```python
from build123d import *

# Parameters (mm, degrees)
FILLET1_R      = 6
CHAMFER1_SIZE  = 1
CHAMFER1_SIZE2 = 2
CHAMFER2_SIZE  = 0.5


with BuildPart() as part:
    # Sketch1 → Revolve1 (revolve)
    with BuildSketch(Plane(origin=(0, 0, 0), x_dir=(0, 0, -1), z_dir=(1, 0, 0)), mode=Mode.PRIVATE) as revolve1_sk:
        Polygon((0, 0), (0, -78.067128988), (11, -78.067128988), (11, -75.067128988), (2.5, -75.067128988), (2.5, -8), (1.5, -8), (1.5, -3), (2.5, -3), (2.5, 0), align=None)
    revolve(revolve1_sk.sketch.rotate(Axis((0, 0, 0), (0, -1, 0)), 180), axis=Axis((0, 0, 0), (0, -1, 0)))

    # Fillet1
    fillet1_edges = [part.edges().sort_by_distance(p)[0] for p in [
        (0, -75.067128988, -2.5),
    ]]
    fillet(fillet1_edges, radius=FILLET1_R)

    # Chamfer1
    chamfer1_edges = [part.edges().sort_by_distance(p)[0] for p in [
        (0, -75.067128988, -11),
    ]]
    chamfer1_side = [part.faces().sort_by_distance(p)[0] for p in [
        (0, -76.567128988, -11),
    ]]
    chamfer(chamfer1_edges, length=CHAMFER1_SIZE, length2=CHAMFER1_SIZE2, reference=chamfer1_side[0])

    # Chamfer2
    chamfer2_edges = [part.edges().sort_by_distance(p)[0] for p in [
        (0, 0, -2.5),
    ]]
    chamfer(chamfer2_edges, length=CHAMFER2_SIZE)


solid = part.part
```
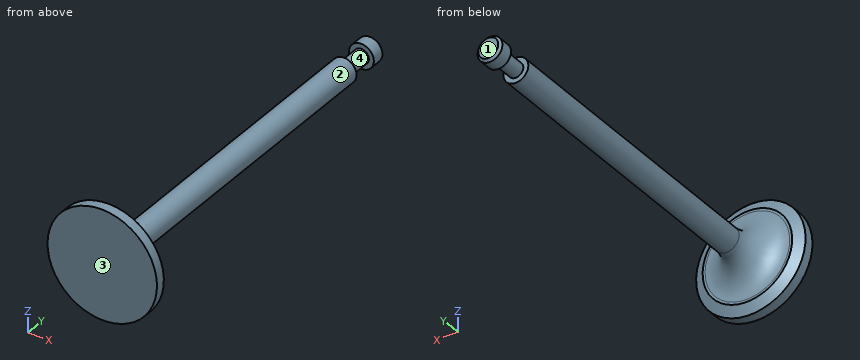
Build history of the part. All positions in model axes, mm. Face numbers are marked on the shaded views. Give positions to 0.01 mm unless a question says otherwise; leave off trailing zeros. Loops run counter-clockwise (first coordinate to the right, second up) from the corner with the lowest first, then second, coordinate; pieces in that order, holes last. Notation, with made-up numbers: (50.5, 36) - (85.5, 36) arc R21 ccw to (85.5, 75) - close; hole circle Ø10 at (58, 12). An arc over 180 degrees is marked (long way). Use a Markdown table: item, result.
(1) Band-saw the part on C-C (y = -50). Give the cut face in (x, z), and give its area (3 significant figures).
Taken from the geometry:
| item | result |
|---|---|
| outline | circle Ø5 at (0, 0) |
| area | 19.6 mm2 |
(2) Band-saw the part on A-A (z = 0). Give the cut face in (x, y), and give its area (3 significant figures).
Taken from the geometry:
| item | result |
|---|---|
| outline | (-11, -78.07) - (11, -78.07) - (11, -76.07) - (9, -75.07) - (8.5, -75.07) arc R6 cw to (2.5, -69.07) - (2.5, -8) - (1.5, -8) - (1.5, -3) - (2.5, -3) - (2.5, -0.5) - (2, 0) - (-2, 0) - (-2.5, -0.5) - (-2.5, -3) - (-1.5, -3) - (-1.5, -8) - (-2.5, -8) - (-2.5, -69.07) arc R6 cw to (-8.5, -75.07) - (-9, -75.07) - (-11, -76.07) - close |
| area | 445 mm2 |
(3) Drop flat-ended pins along their axis: pin 1 Ø12 at (y, z) = (-27.5, 7.5) entering from +X; pin 2 Ø6 at (x, y) = (1.5, -12) entering from +Z; pin 3 Ø4 at (x, y) = (-5, -64.5) entering from +Z; pin 4 Ø10 at (x, z) = (-7, -7) entering from +Y. Give the stop position or say it passes through.
Taken from the geometry:
| item | result |
|---|---|
| pin 1 | x = 2 |
| pin 2 | z = 2.5 |
| pin 3 | through |
| pin 4 | y = -73.87 |
(4) Wall check: line 1 along Y through (x, z) = (0.5, 8.25); line 2 along X through (y, z) = (-9.5, -0.25); line 3 along Y through (x, z) = (-4.25, 6.75). Give the ranges that are in metal, low to high.
Taken from the geometry:
| item | result |
|---|---|
| line 1 | -78.07 to -75.06 |
| line 2 | -2.49 to 2.49 |
| line 3 | -78.07 to -75.04 |
(5) Band-saw the part on B-B (x = 0). Give the cut face in (y, z), and give its area (3 significant figures).
Taken from the geometry:
| item | result |
|---|---|
| outline | (-78.07, -11) - (-76.07, -11) - (-75.07, -9) - (-75.07, -8.5) arc R6 cw to (-69.07, -2.5) - (-8, -2.5) - (-8, -1.5) - (-3, -1.5) - (-3, -2.5) - (-0.5, -2.5) - (0, -2) - (0, 2) - (-0.5, 2.5) - (-3, 2.5) - (-3, 1.5) - (-8, 1.5) - (-8, 2.5) - (-69.07, 2.5) arc R6 cw to (-75.07, 8.5) - (-75.07, 9) - (-76.07, 11) - (-78.07, 11) - close |
| area | 445 mm2 |
(6) Pull direction Y, two halves, no side cores. Call the marked faces 1, 2, 3 and 4: +Y half, -Y half, draft (parallel to the pull), parting line (faces both ways), or undercut.
Taken from the geometry:
| item | result |
|---|---|
| face 1 | +Y half |
| face 2 | draft |
| face 3 | -Y half |
| face 4 | undercut |
